The listing builds one solid part. Answer for the finished solid, in the listing's coordinates (mm). Face numbers are marked on the shaded views. A direction names the side the tool comes from. Coordinates: 2 decimals unless noted, no trailing zeros. Order: outer loops, then holes, each group sorted by start corner. A loop starts at its lowest first (then second) coordinate and runs counter-clockwise, first axis right, second up. Notation, with made-up numbers: (19, 76) - (55, 76) arc R23 ccw to (55, 94) - close; hole circle Ø6 at (35, -2.5). An arc over 180 degrees is marked (long way). Use a Markdown table: item, result. Add a question column.
Item 1: The part is cut by section A-A, the plane x = 21. Give the vertices of the cut face in (y, z).
Item 2: The mould has two halves that part along X. Classify the marked faces 1, 2 and 3: released by +X, released by -X, zero draft, split by the parting line, or undercut.
Item 3: The part is cut by section C-C, the plane x = 0. Give the vertices of the cut face in (y, z), then the cut area to 3 significant figures.
Item 4: The part is cut by section D-D, the plane x = -35. Give the vertices of the cut face in (y, z), then the cut area to 3 significant figures.
Item 5: The part is cut by section B-B, the plane y = 0. Give the vertices of the cut face in (x, z), then the cut area to 3 significant figures.
Item 6: Find the intervals of material crossed by line 1 along X through (y, z) = (-3, 257); line 2 along Z through (x, y) = (-33, -33.5); line 3 along Z through (x, y) = (-34, 70.5), in increasing order.
Item 7: Flat-ended cylindrical pins translate along their axes: P1, Ø3, axis at y = 0.5, z = 241, coming from the +X side; P2, Ø12, axis at x = 57, y = -45.5, coming from the +Z side; P3, Ø3, axis at y = -27.5, z = 148.5, coming from the -X side; P4, Ø2, axis at x = -54, y = 59, coming from the -Z side. Find the tip coordinate at first contact, or state that the pin passes through.
Item 8: For the marked faces 4, 5, 6, 7 and 8, determine the directions among +Z, -Z, +X, -X, +Y, -Y from which every point of the face is accessible in a straight line to the end or side of a thin tool.
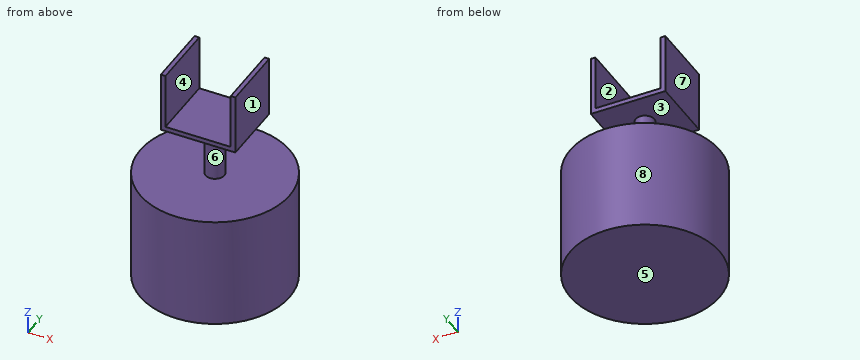
from build123d import *

# Parameters (mm, degrees)
F0_R     = 101.6
F1_DEPTH = 152.4
F2_R     = 12.7
F3_DEPTH = 76.2
F4_W     = 101.6
F4_H     = 88.9
F4_R     = 12.7
F5_DEPTH = 6.35
F6_W     = 6.35
F6_H     = 88.9
F7_DEPTH = 76.2


# Not quite as in the source:
# - a feature names something its author has since deleted; it is built from what else it names


with BuildPart() as f1:
    # F0 (on Top) → F1 (new body)
    with BuildSketch(Plane.XY):
        Circle(F0_R)
    extrude(amount=F1_DEPTH)

    # F2 (on face) → F3 (join)
    with BuildSketch(Plane.XY.offset(152.4)):
        Circle(F2_R)
    extrude(amount=F3_DEPTH)

    # F4 (on face) → F5 (join)
    with BuildSketch(Plane.XY.offset(228.6)):
        Rectangle(F4_W, F4_H)
        Circle(F4_R, mode=Mode.SUBTRACT)
        Circle(F4_R)
    extrude(amount=F5_DEPTH)

    # F6 (on face) → F7 (join)
    with BuildSketch(Plane.XY.offset(234.95)):
        with Locations((-47.625, 0)):
            Rectangle(F6_W, F6_H)
        with Locations((47.625, 0)):
            Rectangle(F6_W, F6_H)
    extrude(amount=F7_DEPTH)


solid = f1.part
Solution:
| question | item | result |
|---|---|---|
| 1 | outline | (-99.41, 0) - (99.41, 0) - (99.41, 152.4) - (-99.41, 152.4) - close; (-44.45, 228.6) - (44.45, 228.6) - (44.45, 234.95) - (-44.45, 234.95) - close |
| 2 | face 1 | released by +X |
| 2 | face 2 | undercut |
| 2 | face 3 | zero draft |
| 3 | outline | (-101.6, 0) - (101.6, 0) - (101.6, 152.4) - (12.7, 152.4) - (12.7, 228.6) - (44.45, 228.6) - (44.45, 234.95) - (-44.45, 234.95) - (-44.45, 228.6) - (-12.7, 228.6) - (-12.7, 152.4) - (-101.6, 152.4) - close |
| 3 | area | 33,500 mm2 |
| 4 | outline | (-95.38, 0) - (95.38, 0) - (95.38, 152.4) - (-95.38, 152.4) - close; (-44.45, 228.6) - (44.45, 228.6) - (44.45, 234.95) - (-44.45, 234.95) - close |
| 4 | area | 29,600 mm2 |
| 5 | outline | (-101.6, 0) - (101.6, 0) - (101.6, 152.4) - (12.7, 152.4) - (12.7, 228.6) - (50.8, 228.6) - (50.8, 311.15) - (44.45, 311.15) - (44.45, 234.95) - (-44.45, 234.95) - (-44.45, 311.15) - (-50.8, 311.15) - (-50.8, 228.6) - (-12.7, 228.6) - (-12.7, 152.4) - (-101.6, 152.4) - close |
| 5 | area | 34,500 mm2 |
| 6 | line 1 | x = -50.8 to -44.45, 44.45 to 50.8 |
| 6 | line 2 | z = 0 to 152.4, 228.6 to 234.95 |
| 6 | line 3 | z = 0 to 152.4 |
| 7 | P1 | stops at x = 50.8 |
| 7 | P2 | stops at z = 152.4 |
| 7 | P3 | stops at x = -98.22 |
| 7 | P4 | stops at z = 0 |
| 8 | face 4 | +Z, +Y, -Y |
| 8 | face 5 | -Z, +X, -X, +Y, -Y |
| 8 | face 6 | none |
| 8 | face 7 | +Z, -X, +Y, -Y |
| 8 | face 8 | +Z, -Z |
